Design review of the part built by this model. Coordinates are the model's own, in mm. Coordinates: 2 decimals unless noted, no trailing zeros. Write each loop counter-clockwise with the first axis right and the second up, starting at its lowest first coordinate (ties: lowest second). Pieces come first, ordered by that corner, then holes. Notation, with made-up numbers: M 76,6.25 L 95,6.25 A27 ccw 95,40.25 Z; hole C 27.25,34.5 d6. An arc over 180 degrees is marked long. Write each question's results on one line, items separated by ' | '. Start each with the question number.
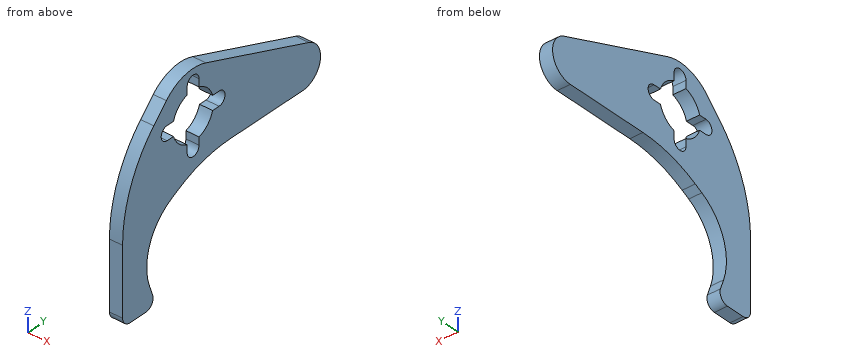
```python
from build123d import *

# Parameters (mm, degrees)
PAD054_DEPTH = 3
FILLET009_R  = 2
FILLET010_R  = 30


with BuildPart() as part:
    # Sketch105 → Pad054 (new body)
    with BuildSketch(Plane.YZ):
        with BuildLine():
            Line((-19, -34.775252), (-19, -5.310494))
            Line((-19, -5.310494), (-7.202157, 6.937502))
            ThreePointArc((3.420201, 9.396926), (-2.255657, 9.74228), (-7.202157, 6.937502))
            Line((3.420201, 9.396926), (31.182699, -0.707796))
            ThreePointArc((29.544233, -10), (34.262008, -6.041316), (31.182699, -0.707796))
            Line((29.544233, -10), (2.5, -10))
            Line((2.5, -10), (-5.882353, -14.470588))
            ThreePointArc((-5.882353, -14.470588), (-11.672587, -21.027783), (-11.746158, -29.775252))
            Line((-11.746158, -29.775252), (-9.926307, -34.775252))
            Line((-19, -34.775252), (-9.926307, -34.775252))
        make_face()
        with BuildLine():
            ThreePointArc((-7, 1.6), (-8.6, 0), (-7, -1.6))
            Line((-7, -1.6), (-5.262129, -1.6))
            ThreePointArc((-5.262129, -1.6), (-3.889087, -3.889087), (-1.6, -5.262129))
            Line((-1.6, -7), (-1.6, -5.262129))
            ThreePointArc((-1.6, -7), (0, -8.6), (1.6, -7))
            Line((1.6, -7), (1.6, -5.262129))
            ThreePointArc((1.6, -5.262129), (3.889087, -3.889087), (5.262129, -1.6))
            Line((5.262129, -1.6), (7, -1.6))
            ThreePointArc((7, -1.6), (8.6, 0), (7, 1.6))
            Line((7, 1.6), (5.262129, 1.6))
            ThreePointArc((5.262129, 1.6), (3.889087, 3.889087), (1.6, 5.262129))
            Line((1.6, 7), (1.6, 5.262129))
            ThreePointArc((1.6, 7), (0, 8.6), (-1.6, 7))
            Line((-1.6, 7), (-1.6, 5.262129))
            ThreePointArc((-1.6, 5.262129), (-3.889087, 3.889087), (-5.262129, 1.6))
            Line((-7, 1.6), (-5.262129, 1.6))
        make_face(mode=Mode.SUBTRACT)
    extrude(amount=PAD054_DEPTH)

    # Fillet009
    fillet009_edges = [part.edges().sort_by_distance(p)[0] for p in [
        (1.5, -9.926307, -34.775252),
        (1.5, -19, -34.775252),
    ]]
    fillet(fillet009_edges, radius=FILLET009_R)

    # Fillet010
    fillet010_edges = [part.edges().sort_by_distance(p)[0] for p in [
        (1.5, -19, -5.310494),
        (1.5, 2.5, -10),
    ]]
    fillet(fillet010_edges, radius=FILLET010_R)


solid = part.part
```
Item 1: Insertion check: pin 1 Ø8 at (y, z) = (-2, -19.5) entering from -X; pin 2 Ø0.9 at (x, y) = (1, -6) entering from -Z; pin 3 Ø0.9 at (x, y) = (2, 6) entering from +Z; pin 4 Ø6 at (y, z) = (7, -11.5) entering from +X. Each pin has a flat end and moves straight along its axis. Give the tip position at first contact, or say it passes through.
Item 2: We need section D-D on z = -18. State the section outline as (x, y) points.
Item 3: Wall thickness on L1, parallel to Y at x = 2.8, z = -6.5; L2, parallel to Z at x = 1.8, y = 21; L3, parallel to Z at x = 1.8, y = -5.5: over which ranges is each line inside the solid? List them lowest first.
Item 4: We need section B-B on z = 0. State the section outline as (x, y) points.
Item 5: We need section C-C on y = 0. State the section outline as (x, z) points.
Answer:
1) pin 1: passes through | pin 2: stops at z = -14.79 | pin 3: stops at z = 8.62 | pin 4: stops at x = 3
2) outline: M 0,-19 L 3,-19 L 3,-10 L 0,-10 Z
3) L1: y = -16.95 to -1.6, 1.6 to 34.16 | L2: z = -10 to 3 | L3: z = -14.27 to -1.6, 1.6 to 8.35
4) outline: M 0,-13.43 L 3,-13.43 L 3,-8.6 L 0,-8.6 Z; M 0,8.6 L 3,8.6 L 3,29.24 L 0,29.24 Z
5) outline: M 0,-11.72 L 3,-11.72 L 3,-8.6 L 0,-8.6 Z; M 0,8.6 L 3,8.6 L 3,10 L 0,10 Z
